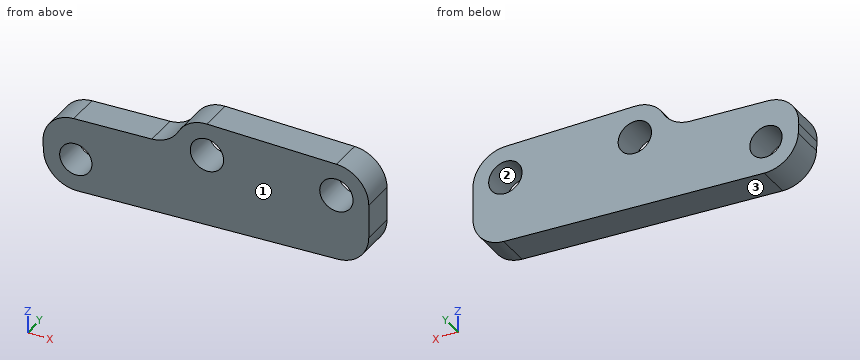
from build123d import *

# Parameters (mm, degrees)
F1_DEPTH = 25.4
F3_D     = 26.1874
F4_R     = 25.4
F7_D     = 25.3492


# Not quite as in the source:
# - a feature names something its author has since deleted; it is built from what else it names


with BuildPart() as f1:
    # F0 (on Front) → F1 (new body)
    with BuildSketch(Plane.XZ):
        Polygon((-177.8, -25.4), (76.2, -12.7), (-76.2, -12.7), (-76.2, 12.7), (-76.2, 38.1), (-180.7137157107, 32.8743142145), align=None)
        Polygon((-76.2, -12.7), (76.2, -12.7), (76.2, 12.7), (50.8, 12.7), (-50.7999999312, 12.7), (-76.2, 12.7), align=None)
        with BuildLine():
            Line((50.8, 12.7), (76.2, 12.7))
            Line((76.2, 12.7), (76.2, 38.1))
            ThreePointArc((76.2, 38.1), (68.7605122421, 20.1394877579), (50.8, 12.7))
        make_face()
        with BuildLine():
            Line((-76.2, 38.1), (-76.2, 12.7))
            Line((-76.2, 12.7), (-50.7999999312, 12.7))
            ThreePointArc((-50.7999999312, 12.7), (-68.7605122178, 20.1394877335), (-76.2, 38.1))
        make_face()
        with BuildLine():
            Line((-50.7999999312, 12.7), (50.8, 12.7))
            ThreePointArc((50.8, 12.7), (25.4, 38.1), (50.8, 63.5))
            Line((50.8, 63.5), (-50.8, 63.5))
            ThreePointArc((-50.8, 63.5), (-32.8394877579, 56.0605122421), (-25.4, 38.1))
            ThreePointArc((-25.4, 38.1), (-32.8394877335, 20.1394877822), (-50.7999999312, 12.7))
        make_face()
        with BuildLine():
            ThreePointArc((50.8, 63.5), (25.4, 38.1), (50.8, 12.7))
            ThreePointArc((50.8, 12.7), (68.7605122421, 20.1394877579), (76.2, 38.1))
            ThreePointArc((76.2, 38.1), (68.7605122421, 56.0605122421), (50.8, 63.5))
        make_face()
        with BuildLine():
            ThreePointArc((-76.2, 38.1), (-68.7605122178, 20.1394877335), (-50.7999999312, 12.7))
            ThreePointArc((-50.7999999312, 12.7), (-32.8394877335, 20.1394877822), (-25.4, 38.1))
            ThreePointArc((-25.4, 38.1), (-32.8394877579, 56.0605122421), (-50.8, 63.5))
            ThreePointArc((-50.8, 63.5), (-68.7605122421, 56.0605122421), (-76.2, 38.1))
        make_face()
    extrude(amount=F1_DEPTH)

    # F3 (through all)
    with Locations(Plane.XZ.offset(25.4)):
        with Locations((-50.8, 38.1), (50.8, 38.1)):
            Hole(F3_D / 2)

    # F4
    f4_edges = [f1.edges().sort_by_distance(p)[0] for p in [
        (76.2, -12.7, -12.7),
        (-177.8, -12.7, -25.4),
        (-76.2, -12.7, 38.1),
        (-180.713716, -12.7, 32.874314),
    ]]
    fillet(f4_edges, radius=F4_R)

    # F7 (through all)
    with Locations(Plane.XZ.offset(25.4)):
        with Locations((-153.7001060629, 1.2367248779)):
            Hole(F7_D / 2)


solid = f1.part
CAD build for the part. Positions are in the model's coordinates, mm. Face numbers are marked on the shaded views. Round coordinates to 2 decimals unless told otherwise and drop trailing zeros. Loops run counter-clockwise (first coordinate to the right, second up) from the corner with the lowest first, then second, coordinate; pieces in that order, holes last.
(1) Wall check: line 1 along X through (y, z) = (-12.5, 42); line 2 along X through (y, z) = (-13.5, 27); line 3 along Z through (x, y) = (50.8, -16). Give the ranges that are in metal, low to high.
(2) Drop flat-ended pins along their axis: pin 1 (8 mm diameter, centred on y = -3.5, z = 44.5, fed in from -X); pin 2 (23.5 mm diameter, centred on x = -50.8, z = 38.1, fed in from -Y); pin 3 (2 mm diameter, centred on x = -6, y = -10.5, fed in from -Z); pin 4 (1 mm diameter, centred on x = 1, y = -11, fed in from -Z) (3 decimals). Give the stop position or say it passes through.
(3) Cut at C-C (y = -4.25). Give the cut face in (x, z).
(4) Cut at A-A (z = -5). Give the cut face in (x, y), plus the area to 3 significant figures.
(5) Two-plate mould, pull along X, no slides. Class the marked faces 1, 2 and 3: +X half, -X half, draft (parallel to the pull), parting line (faces both ways), or undercut.
(6) Cut at B-B (x = 56.5). Give the cut face in (y, z), plus the area to 3 significant figures.
(7) Cut at D-D (x = -106). Give the cut face in (y, z).
Findings below:
1. line 1: x = -80.42 to -63.3, -38.3 to 38.3, 63.3 to 75.9
1. line 2: x = -171.77 to -57.75, -43.85 to 43.85, 57.75 to 76.2
1. line 3: z = -13.97 to 25.01, 51.19 to 63.5
2. pin 1: stops at x = -82.75
2. pin 2: passes through
2. pin 3: stops at z = -16.86
2. pin 4: stops at z = -16.485
3. outline: (-179.45, 7.51) - (-179.07, -0.03) arc R25.4 ccw to (-152.43, -24.13) - (52.07, -13.91) arc R25.4 ccw to (76.2, 11.46) - (76.2, 38.1) arc R25.4 ccw to (50.8, 63.5) - (-50.8, 63.5) arc R25.4 ccw to (-73.06, 50.34) arc R25.4 cw to (-94.05, 37.21) - (-155.35, 34.14) arc R25.4 ccw to start; hole circle Ø25.35 at (-153.7, 1.24); hole circle Ø26.19 at (-50.8, 38.1); hole circle Ø26.19 at (50.8, 38.1)
4. outline: (-178.32, -25.4) - (-164.73, -25.4) - (-164.73, 0) - (-178.32, 0) - close; (-142.67, -25.4) - (70.14, -25.4) - (70.14, 0) - (-142.67, 0) - close
4. area: 5,750 mm2
5. face 1: draft
5. face 2: undercut
5. face 3: +X half
6. outline: (-25.4, -13.29) - (0, -13.29) - (0, 26.31) - (-25.4, 26.31) - close; (-25.4, 49.89) - (0, 49.89) - (0, 62.85) - (-25.4, 62.85) - close
6. area: 1,340 mm2
7. outline: (-25.4, -21.81) - (0, -21.81) - (0, 36.61) - (-25.4, 36.61) - close
